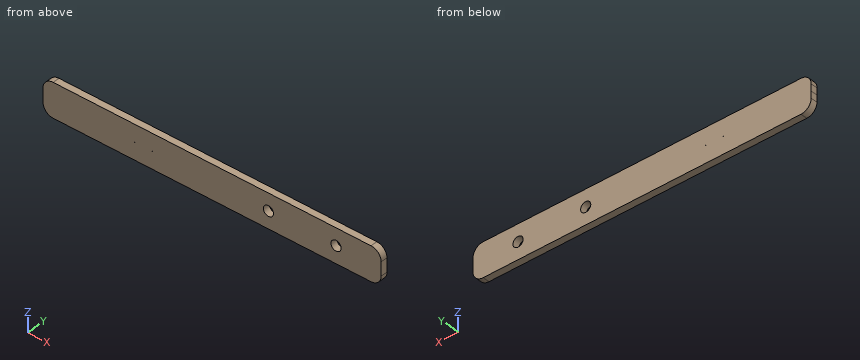
from build123d import *

# Parameters (mm, degrees)
SKETCH1_W             = 100
SKETCH1_H             = 10
BOSS_EXTRUDE1_DEPTH   = 2
FILLET1_R             = 3
F_3_0MM_DOWEL_HOLE1_D = 3
SKETCH2_W             = 47
SKETCH2_H             = 0.001
CUT_EXTRUDE1_DEPTH    = 10


with BuildPart() as part:
    # Sketch1 → Boss-Extrude1 (new body)
    with BuildSketch(Plane(origin=(0, 0, 0), x_dir=(1, 0, 0), z_dir=(0, 1, 0))):
        Rectangle(SKETCH1_W, SKETCH1_H)
    extrude(amount=BOSS_EXTRUDE1_DEPTH)

    # Fillet1
    fillet1_edges = [part.edges().sort_by_distance(p)[0] for p in [
        (50, 1, 5),
        (-50, 1, 5),
        (-50, 1, -5),
        (50, 1, -5),
    ]]
    fillet(fillet1_edges, radius=FILLET1_R)

    # Ø3.0mm Dowel Hole1 (through all)
    with Locations(Plane(origin=(0, 2, 0), x_dir=(1, 0, 0), z_dir=(0, 1, 0))):
        with Locations((36.669467955, 0), (16.669467955, 0)):
            Hole(F_3_0MM_DOWEL_HOLE1_D / 2)

    # Sketch2 → Cut-Extrude1 (cut)
    with BuildSketch(Plane(origin=(0, 2, 0), x_dir=(1, 0, 0), z_dir=(0, 1, 0))):
        with Locations((-26.5, 0)):
            Rectangle(SKETCH2_W, SKETCH2_H)
    extrude(amount=-CUT_EXTRUDE1_DEPTH, mode=Mode.SUBTRACT)


solid = part.part
Source: CAD feature listing. Evaluate the final solid. Frame: model axes, mm. Coordinates: 2 decimals unless noted, no trailing zeros. Answer in a Markdown table with one row per item. Add a question column.
Q1. Section A-A on y = 0.7. Give the number of separate pieces and of enclosed holes in the cut face, and give its area (3 significant figures).
Q2. Ray query, line 1 along X through (y, z) = (1.35, -1); line 2 along X through (y, z) = (0.1, 2.25); line 3 along X through (y, z) = (1.2, 0.75). Return the intervals inside material, ascending.
Q3. Contact query for a flat-ended pin moving along its axis: pin 1 Ø1 at (x, z) = (-26, 0) entering from -Y. Output: stop coordinate, or through.
Computed values:
| question | item | result |
|---|---|---|
| 1 | separate pieces | 1 |
| 1 | enclosed holes | 2 |
| 1 | area | 978 mm^2 |
| 2 | line 1 | x = -50 to 15.55, 17.79 to 35.55, 37.79 to 50 |
| 2 | line 2 | x = -49.99 to 49.99 |
| 2 | line 3 | x = -50 to 15.37, 17.97 to 35.37, 37.97 to 50 |
| 3 | pin 1 | stops at y = 0 |
